Geometry check sheet. Reference: the model listing, model coordinates, mm. Face numbers are marked on the shaded views. A direction names the side the tool comes from. Give positions to 0.01 mm unless a question says otherwise; leave off trailing zeros. Write item = value, one per line. Start each with the question number.
from build123d import *

# Parameters (mm, degrees)
SKICA1_R                  = 20
P_IDAT_VYSUNUT_M1_DEPTH   = 66
SKICA2_R                  = 27.5
P_IDAT_VYSUNUT_M2_DEPTH   = 35
SKICA3_R                  = 26.5
P_IDAT_VYSUNUT_M3_DEPTH   = 84
SKICA4_R                  = 27.5
P_IDAT_VYSUNUT_M4_DEPTH   = 35
SKICA5_R                  = 20
P_IDAT_VYSUNUT_M5_DEPTH   = 30
SKICA6_R                  = 17.5
P_IDAT_VYSUNUT_M6_DEPTH   = 90
ZKOSEN_3_SIZE             = 6
ZKOSEN_3_SIZE2            = 3.464101615
SKICA9_OUTSIDE_W          = 126.756
SKICA9_OUTSIDE_H          = 126.756
ODEBRAT_VYSUNUT_M16_DEPTH = 90
ZKOSEN_4_SIZE             = 0.5
M10_Z_VIT1_D              = 8.5
M10_Z_VIT1_DEPTH          = 30
M10_Z_VIT1_TIP            = 2.553657631


with BuildPart() as part:
    # Skica1 → Přidat vysunutím1 (new body)
    with BuildSketch(Plane.XY):
        Circle(SKICA1_R)
    extrude(amount=P_IDAT_VYSUNUT_M1_DEPTH)

    # Skica2 → Přidat vysunutím2 (add)
    with BuildSketch(Plane.XY.offset(66)):
        Circle(SKICA2_R)
    extrude(amount=P_IDAT_VYSUNUT_M2_DEPTH)

    # Skica3 → Přidat vysunutím3 (add)
    with BuildSketch(Plane.XY.offset(101)):
        Circle(SKICA3_R)
    extrude(amount=P_IDAT_VYSUNUT_M3_DEPTH)

    # Skica4 → Přidat vysunutím4 (add)
    with BuildSketch(Plane.XY.offset(185)):
        Circle(SKICA4_R)
    extrude(amount=P_IDAT_VYSUNUT_M4_DEPTH)

    # Skica5 → Přidat vysunutím5 (add)
    with BuildSketch(Plane.XY.offset(220)):
        Circle(SKICA5_R)
    extrude(amount=P_IDAT_VYSUNUT_M5_DEPTH)

    # Skica6 → Přidat vysunutím6 (add)
    with BuildSketch(Plane.XY.offset(250)):
        Circle(SKICA6_R)
    extrude(amount=P_IDAT_VYSUNUT_M6_DEPTH)

    # Zkosení3
    zkosen_3_edges = [part.edges().sort_by_distance(p)[0] for p in [
        (-17.5, 0, 340),
    ]]
    zkosen_3_side = [part.faces().sort_by_distance(p)[0] for p in [
        (-17.5, 0, 295),
    ]]
    chamfer(zkosen_3_edges, length=ZKOSEN_3_SIZE, length2=ZKOSEN_3_SIZE2, reference=zkosen_3_side[0])

    # Skica9 outside → Odebrat vysunutím16 (cut)
    with BuildSketch(Plane.XY.offset(340)):
        Rectangle(SKICA9_OUTSIDE_W, SKICA9_OUTSIDE_H)
        with BuildLine():
            Line((-4.25, 14.385322381), (-4.25, 16.976086121))
            ThreePointArc((-4.25, 16.976086121), (0, 17.5), (4.25, 16.976086121))
            Line((4.25, 16.976086121), (4.25, 14.385322381))
            ThreePointArc((4.25, 14.385322381), (7.5, 12.990381057), (10.333054623, 10.873269156))
            Line((10.333054623, 10.873269156), (12.576721838, 12.168651027))
            ThreePointArc((12.576721838, 12.168651027), (15.155444566, 8.75), (16.826721838, 4.807435095))
            Line((16.826721838, 4.807435095), (14.583054623, 3.512053224))
            ThreePointArc((14.583054623, 3.512053224), (15, 0), (14.583054623, -3.512053224))
            Line((14.583054623, -3.512053224), (16.826721838, -4.807435095))
            ThreePointArc((16.826721838, -4.807435095), (15.155444566, -8.75), (12.576721838, -12.168651027))
            Line((12.576721838, -12.168651027), (10.333054623, -10.873269156))
            ThreePointArc((10.333054623, -10.873269156), (7.5, -12.990381057), (4.25, -14.385322381))
            Line((4.25, -14.385322381), (4.25, -16.976086121))
            ThreePointArc((4.25, -16.976086121), (0, -17.5), (-4.25, -16.976086121))
            Line((-4.25, -16.976086121), (-4.25, -14.385322381))
            ThreePointArc((-4.25, -14.385322381), (-7.5, -12.990381057), (-10.333054623, -10.873269156))
            Line((-10.333054623, -10.873269156), (-12.576721838, -12.168651027))
            ThreePointArc((-12.576721838, -12.168651027), (-15.155444566, -8.75), (-16.826721838, -4.807435095))
            Line((-16.826721838, -4.807435095), (-14.583054623, -3.512053224))
            ThreePointArc((-14.583054623, -3.512053224), (-15, 0), (-14.583054623, 3.512053224))
            Line((-14.583054623, 3.512053224), (-16.826721838, 4.807435095))
            ThreePointArc((-16.826721838, 4.807435095), (-15.155444566, 8.75), (-12.576721838, 12.168651027))
            Line((-12.576721838, 12.168651027), (-10.333054623, 10.873269156))
            ThreePointArc((-10.333054623, 10.873269156), (-7.5, 12.990381057), (-4.25, 14.385322381))
        make_face(mode=Mode.SUBTRACT)
    extrude(amount=-ODEBRAT_VYSUNUT_M16_DEPTH, mode=Mode.SUBTRACT)

    # Zkosení4
    zkosen_4_edges = [part.edges().sort_by_distance(p)[0] for p in [
        (-27.5, 0, 185),
        (-27.5, 0, 220),
        (-20, 0, 0),
        (-20, 0, 250),
        (-27.5, 0, 66),
        (-27.5, 0, 101),
    ]]
    chamfer(zkosen_4_edges, length=ZKOSEN_4_SIZE)

    # M10 závit1
    with Locations(Plane(origin=(0, 0, 0), x_dir=(-1, 0, 0), z_dir=(0, 0, -1))):
        with Locations((0, 0)):
            Hole(M10_Z_VIT1_D / 2, depth=M10_Z_VIT1_DEPTH)
            with Locations((0, 0, -(M10_Z_VIT1_DEPTH + M10_Z_VIT1_TIP / 2))):  # 118° drill point
                Cone(0, M10_Z_VIT1_D / 2, M10_Z_VIT1_TIP, mode=Mode.SUBTRACT)


solid = part.part
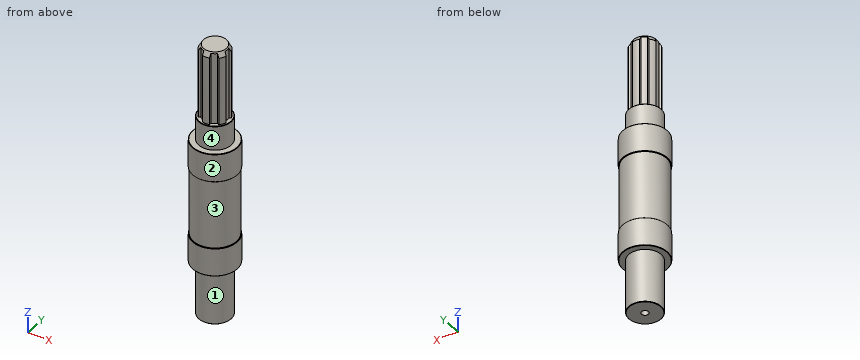
1) Gauge pin test, flat ends, axial feed: P1, Ø12, axis at x = -21, z = 201.5, coming from the +Y side; P2, Ø1, axis at x = -15, y = 10.5, coming from the +Z side; P3, Ø1, axis at x = 11.5, y = 20, coming from the +Z side. Record the tip position at first contact, or that the pin passes through.
2) Release check for a two-part mould opening along Z. For the marked faces 3 and 4 record: pulls with the +Z half, pulls with the -Z half, needs draft (parallel to the pull), parting line crosses it, or undercut.
3) Material ranges on line 1 along Y through (x, z) = (0, 14); line 2 along Y through (x, z) = (5, 201); line 3 along Z through (x, y) = (19, 12.5), recorded low to high.
4) Tool access check on the marked faces 1 and 2. Record the directions out of +Z, -Z, +X, -X, +Y, -Y that give a thin tool (end or side, any length) a straight path to the whole face; none if there is none.
Checked values:
q1.P1 = 23.05
q1.P2 = 250
q1.P3 = 220
q2.face_3 = undercut
q2.face_4 = needs draft
q3.line_1 = -20 to -4.25, 4.25 to 20
q3.line_2 = -27.04 to 27.04
q3.line_3 = 66 to 220
q4.face_1 = -Z
q4.face_2 = +Z, -Z
